from build123d import *

# Parameters (mm, degrees)
CUT_EXTRUDE1_START = -3
CUT_EXTRUDE1_DEPTH = 12
CIRPATTERN1_COUNT  = 25


with BuildPart() as part:
    # Sketch6 → Revolve1 (revolve)
    with BuildSketch(Plane.XY):
        with BuildLine():
            Line((9.75, 22), (10.5, 22))
            Line((10.5, 22), (10.5, 3))
            Line((10.5, 3), (-10.5, 3))
            Line((-10.5, 3), (-10.5, 13))
            Line((-10.5, 13), (-4.5, 13))
            Line((-4.5, 13), (-4.5, 22))
            Line((-4.5, 22), (-3.75, 22))
            ThreePointArc((-3.75, 22), (-3.191538955, 20.805038314), (-3, 19.5))
            Line((-3, 19.5), (9, 19.5))
            ThreePointArc((9, 19.5), (9.191538955, 20.805038314), (9.75, 22))
        make_face()
    revolve(axis=Axis((-10.5, 0, 0), (1, 0, 0)))

    # Sketch3 → Cut-Extrude1 (cut)
    with BuildSketch(Plane(origin=(0, 0, 0), x_dir=(0, 0, -1), z_dir=(1, 0, 0)).offset(CUT_EXTRUDE1_START)):
        with BuildLine():
            Line((-1.325, 19.454931894), (-0.896639329, 18.278020624))
            Line((-0.896639329, 18.278020624), (0.896639329, 18.278020624))
            Line((0.896639329, 18.278020624), (1.325, 19.454931894))
            ThreePointArc((1.325, 19.454931894), (0, 19.5), (-1.325, 19.454931894))
        make_face()
    cut_extrude1 = extrude(amount=CUT_EXTRUDE1_DEPTH, mode=Mode.SUBTRACT)

    # CirPattern1: Cut-Extrude1 ×25 about axis
    cirpattern1_axis = Axis((0, 0, 0), (1, 0, 0))
    for i in range(1, CIRPATTERN1_COUNT):
        add(cut_extrude1.rotate(cirpattern1_axis, i * 360 / CIRPATTERN1_COUNT), mode=Mode.SUBTRACT)


solid = part.part
Work out the finished part from the listing and answer in its coordinate system (mm). A direction names the side the tool comes from. Round coordinates to 2 decimals unless told otherwise and drop trailing zeros. Loops run counter-clockwise (first coordinate to the right, second up) from the corner with the lowest first, then second, coordinate; pieces in that order, holes last. Notation, with made-up numbers: M 87,70.5 L 129,70.5 A22 ccw 129,82.5 Z; hole C 86.5,39.25 d6. An arc over 180 degrees is marked long. One line per question, with ' | ' between items. Start each with the question number.
(1) A tool of negligible diameter and unlimited length cuts with its end or side. For faces 1 (the face through (-4.5, -9.5, -9.5)), 2 (the face through (2.92, 9.78, 15.44)), 3 (the face through (2.916, -18.135, 2.278)), 4 (the face through (-3, 1, -19)), from which of +Z, -Z, +X, -X, +Y, -Y can it reach the whole face along a straight path? Write none if from no direction.
(2) For a pull along Y with two mould halves and no side action, classify faces 5 (the face through (9, 6, -18)), 6 (the face through (-3, 18, -5)), 7 (the face through (3.084, -18.883, 4.865)), 8 (the face through (-3, 1, 19)) as released by +Y, released by -Y, zero draft, split by the parting line, or undercut.
(3) A cutting plane is placed at B-B on x = -8.75. Write down the section's boundary in (y, z), plus the area to 3 significant figures.
(4) Find the intervals of material crossed by line 1 (Z direction, x = -4.75, y = 0); line 2 (X direction, y = -14, z = -3.5); line 3 (Y direction, x = -7, z = -3.5), in increasing order.
(5) Flat-ended cylindrical pins translate along their axes: pin 1 Ø10 at (y, z) = (6.5, 14) entering from -X; pin 2 Ø3 at (x, y) = (6, 12) entering from -Z; pin 3 Ø0.6 at (y, z) = (-17.5, 7) entering from -X; pin 4 Ø10 at (x, y) = (-7, -5) entering from +Z. Find the tip coordinate at first contact, or state that the pin passes through.
(6) A cutting plane is placed at A-A on z = 0. Write down the section's boundary in (x, y).
Geometry check:
1) face 1: -X | face 2: none | face 3: -Y | face 4: -Z
2) face 5: undercut | face 6: zero draft | face 7: released by -Y | face 8: undercut
3) outline: C 0,0 d26; hole C 0,0 d6 | area: 503 mm²
4) line 1: z = -13 to -3, 3 to 13 | line 2: x = -4.5 to 10.5 | line 3: y = -12.52 to 12.52
5) pin 1: stops at x = -10.5 | pin 2: stops at z = -15.72 | pin 3: stops at x = -4.5 | pin 4: stops at z = 21.99
6) outline: M -10.5,-13 L -4.5,-13 L -4.5,-22 L -3.75,-22 A4.54 ccw -3,-19.5 L 9,-19.5 A4.54 ccw 9.75,-22 L 10.5,-22 L 10.5,-3 L -10.5,-3 Z; M -10.5,3 L 10.5,3 L 10.5,22 L 9.75,22 A4.54 ccw 9,19.5 L 9,18.28 L -3,18.28 L -3,19.5 A4.54 ccw -3.75,22 L -4.5,22 L -4.5,13 L -10.5,13 Z
